Part model, mm, in its own coordinate system. Face numbers are marked on the shaded views. A direction names the side the tool comes from. Round coordinates to 2 decimals unless told otherwise and drop trailing zeros. Order: outer loops, then holes, each group sorted by start corner. A loop starts at its lowest first (then second) coordinate and runs counter-clockwise, first axis right, second up. Notation, with made-up numbers: (78.25, -8.5) - (104.25, -8.5) arc R10 ccw to (104.25, -3.5) - close; hole circle Ø11 at (66, -5.75). An arc over 180 degrees is marked (long way). Answer as a JSON object with one key per item and string values.
```python
from build123d import *

# Parameters (mm, degrees)
BOSS_EXTRUDE1_DEPTH = 160
SKETCH2_R           = 15
BOSS_EXTRUDE4_DEPTH = 76
RIB4_REACH          = 187.313
SKETCH5_WALL_W      = 502.626496624
SKETCH5_WALL_H      = 12


with BuildPart() as part:
    # Sketch1 → Boss-Extrude1 (new body)
    with BuildSketch(Plane(origin=(0, 0, 0), x_dir=(0, 0, -1), z_dir=(1, 0, 0))):
        Polygon((-26, 5), (26, 5), (26, -5), (50, -5), (50, 7), (38, 7), (38, 19), (-38, 19), (-38, 7), (-50, 7), (-50, -5), (-26, -5), align=None)
    extrude(amount=-BOSS_EXTRUDE1_DEPTH)

    # Sketch2 → Boss-Extrude4 (add)
    with BuildSketch(Plane(origin=(0, 0, -38), x_dir=(-1, 0, 0), z_dir=(0, 0, -1))):
        with BuildLine():
            Line((160, 19), (160, 49))
            ThreePointArc((160, 49), (130, 79), (100, 49))
            Line((100, 49), (100, 19))
            Line((100, 19), (160, 19))
        make_face()
        with Locations((130, 49)):
            Circle(SKETCH2_R, mode=Mode.SUBTRACT)
    extrude(amount=-BOSS_EXTRUDE4_DEPTH)

    # Sketch5 wall → Rib4 (add, up to next)
    with BuildSketch(Plane(origin=(-58.426966292, 47.483146068, 0), x_dir=(-0.898876404493, 0.438202247193, 0), z_dir=(-0.438202247193, -0.898876404493, 0)), mode=Mode.PRIVATE) as rib4_sk1:
        Rectangle(SKETCH5_WALL_W, SKETCH5_WALL_H)
    rib4_tool1 = extrude(rib4_sk1.sketch, amount=RIB4_REACH, mode=Mode.PRIVATE) - part.part
    add(rib4_tool1.solids().sort_by_distance((-58.426966292, 47.483146068, 0))[0])


solid = part.part
```
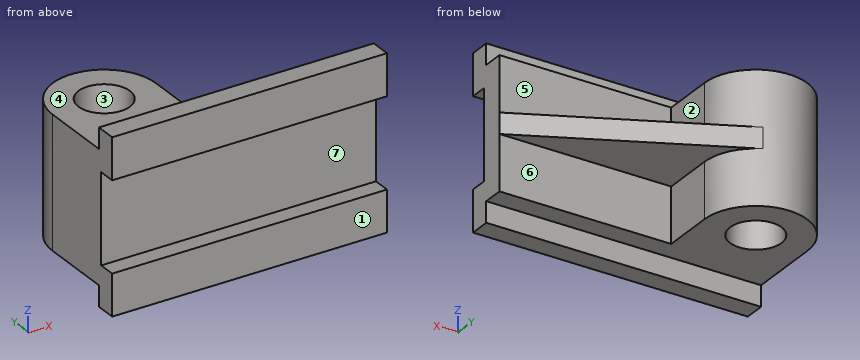
Item 1: Cut at B-B (z = -33). Write the cut outline in (x, y), plus the area to 3 significant figures.
Taken from the geometry:
{"outline": "(-160, -5) - (0, -5) - (0, 19) - (-100, 19) - (-100, 49) arc R30 ccw to (-160, 49) - close; hole circle Ø30 at (-130, 49)", "area": "6,350 mm2"}
Item 2: Two-plate mould, pull along X, no slides. Class the marked faces 1, 2 and 3: pulls with the +X half, pulls with the -X half, needs draft (parallel to the pull), parting line crosses it, or undercut.
Taken from the geometry:
{"face 1": "needs draft", "face 2": "pulls with the +X half", "face 3": "undercut"}
Item 3: Cut at A-A (x = -130). Write the cut outline in (y, z), plus the area to 3 significant figures.
Taken from the geometry:
{"outline": "(-5, -50) - (7, -50) - (7, -38) - (34, -38) - (34, 38) - (7, 38) - (7, 50) - (-5, 50) - (-5, 26) - (5, 26) - (5, -26) - (-5, -26) - close; (64, -38) - (79, -38) - (79, 38) - (64, 38) - close", "area": "3,870 mm2"}
Item 4: Drop flat-ended pins along their axis: P1, Ø2, axis at x = -43, y = 33, coming from the -Z side; P2, Ø1.5, axis at x = -36, z = 7.5, coming from the -Y side; P3, Ø9.5, axis at x = -66.5, z = -18, coming from the +Y side. Give the stop position or say it passes through.
Taken from the geometry:
{"P1": "z = -6", "P2": "y = 5", "P3": "y = 19"}
Item 5: Tool access for the marked faces 4, 5, 6 and 7: list every direction of +Z, -Z, +X, -X, +Y, -Y with a clear straight run to the whole face (end or side of a thin tool).
Taken from the geometry:
{"face 4": "+Z, +X, -X, +Y", "face 5": "+Z, +X, +Y", "face 6": "-Z, +X, +Y", "face 7": "+X, -X, -Y"}
Item 6: Cut at D-D (z = 20). Write the cut outline in (x, y), plus the area to 3 significant figures.
Taken from the geometry:
{"outline": "(-160, 5) - (0, 5) - (0, 19) - (-100, 19) - (-100, 49) arc R30 ccw to (-160, 49) - close; hole circle Ø30 at (-130, 49)", "area": "4,750 mm2"}
Item 7: Probe L1, parallel to Y at x = -130, z = -7; L2, parallel to Y at x = -108.5, z = 40.5; L3, parallel to Z at x = -136, y = 22. List the from-to ranges inside material, lowest first. Write a range as from..to.
Taken from the geometry:
{"L1": "5..34, 64..79", "L2": "-5..7", "L3": "-38..38"}
Item 8: Cut at C-C (y = 61.5). Write the cut outline in (x, z).
Taken from the geometry:
{"outline": "(-157.27, -38) - (-138.29, -38) - (-138.29, 38) - (-157.27, 38) - close; (-121.71, -38) - (-102.73, -38) - (-102.73, -6) - (-87.18, -6) - (-87.18, 6) - (-102.73, 6) - (-102.73, 38) - (-121.71, 38) - close"}
